from build123d import *

# Parameters (mm, degrees)
F0_W     = 25
F0_H     = 25
F1_DEPTH = 25
F2_W     = 8
F2_H     = 3
F3_DEPTH = 25
F4_W     = 20
F4_H     = 5
F5_DEPTH = 3
F7_DEPTH = 1


with BuildPart() as f1:
    # F0 (on Top) → F1 (new body)
    with BuildSketch(Plane.XY):
        Rectangle(F0_W, F0_H)
    extrude(amount=F1_DEPTH)

    # F2 (on face) → F3 (join)
    with BuildSketch(Plane.XY.offset(25)):
        with Locations((6.7, -1.5)):
            Rectangle(F2_W, F2_H)
        with Locations((-6.7, -1.5)):
            Rectangle(F2_W, F2_H)
    extrude(amount=F3_DEPTH)

    # F4 (on face) → F5 (cut)
    with BuildSketch(Plane.XZ.offset(12.5)):
        with Locations((0, 4.7)):
            Rectangle(F4_W, F4_H)
    extrude(amount=-F5_DEPTH, mode=Mode.SUBTRACT)

    # F6 (on face) → F7 (join)
    with BuildSketch(Plane.XZ.offset(12.5)):
        with BuildLine():
            add(Edge.make_bspline(
                [(-6.6, 15.000625), (-4.434936, 15.000625), (-5.517468, 18.000625), (-6.6, 21.000625), (-7.682532, 18.000625), (-8.765064, 15.000625), (-6.6, 15.000625)],
                knots=[0, 0, 0, 2.094395, 2.094395, 4.18879, 4.18879, 6.283185, 6.283185, 6.283185], degree=2, weights=[1, 0.5, 1, 0.5, 1, 0.5, 1]))
        make_face()
        with BuildLine():
            add(Edge.make_bspline(
                [(6.6, 15.000625), (8.765064, 15.000625), (7.682532, 18.000625), (6.6, 21.000625), (5.517468, 18.000625), (4.434936, 15.000625), (6.6, 15.000625)],
                knots=[0, 0, 0, 2.094395, 2.094395, 4.18879, 4.18879, 6.283185, 6.283185, 6.283185], degree=2, weights=[1, 0.5, 1, 0.5, 1, 0.5, 1]))
        make_face()
    extrude(amount=F7_DEPTH)


solid = f1.part
Source: CAD feature listing. Evaluate the final solid. Frame: model axes, mm. A direction names the side the tool comes from. Round coordinates to 2 decimals unless told otherwise and drop trailing zeros. Loops run counter-clockwise (first coordinate to the right, second up) from the corner with the lowest first, then second, coordinate; pieces in that order, holes last. Notation, with made-up numbers: M 8,69.5 L 52,69.5 A29 cw 52,104.5 Z; hole C -30,41.5 d10. An arc over 180 degrees is marked long. Return JSON: item names as keys, results as strings. Group by question number.
1. Section query B-B on z = 31.5. Output: boundary loops of the cut face in (x, y), and give its area (3 significant figures).
2. Section query A-A on x = -1.5. Output: boundary loops of the cut face in (y, z).
3. Mould query, pull axis Z, two halves, no side actions, for faces 5 (the face through (10, -11, 5)), 6 (the face through (-10.7, -2, 37)), 7 (the face through (0, -11, 7.2)), 8 (the face through (7, -1, 50)). Classes: released by +Z, released by -Z, zero draft, split by the parting line, or undercut.
4. Reachability of faces 1 (the face through (0, -9.5, 5)), 2 (the face through (2.7, -2, 37)), 3 (the face through (7, -3, 37)), 4 (the face through (7, 0, 37)) from +Z, -Z, +X, -X, +Y, -Y: full face, straight path, thin tool, end or side. Return the list, or none.
5. Section query D-D on z = 6. Output: boundary loops of the cut face in (x, y).
6. Pin query (flat end, axial travel): pin 1 (0.9 mm diameter, centred on x = 3.5, y = -11.5, fed in from -Z); pin 2 (3.5 mm diameter, centred on x = 2, y = -11.5, fed in from +Z); pin 3 (4 mm diameter, centred on x = -10, z = 44.5, fed in from -Y); pin 4 (2.5 mm diameter, centred on x = -7, z = 40.5, fed in from +Y). Return the tip coordinate at first contact, or that it passes through.
7. Material intervals for line 1 along X through (y, z) = (-2, 39); line 2 along Z through (x, y) = (3.5, -4.75); line 3 along Y through (x, z) = (-1.75, 13), sorted ascending. Write a range as from..to.
8. Section query C-C on y = -1.25. Output: boundary loops of the cut face in (x, z), and give its area (4 significant figures).
Checks:
{
 "1": {"outline": "M -10.7,-3 L -2.7,-3 L -2.7,0 L -10.7,0 Z; M 2.7,-3 L 10.7,-3 L 10.7,0 L 2.7,0 Z", "area": "48.0 mm²"},
 "2": {"outline": "M -12.5,0 L 12.5,0 L 12.5,25 L -12.5,25 L -12.5,7.2 L -9.5,7.2 L -9.5,2.2 L -12.5,2.2 Z"},
 "3": {"face 5": "undercut", "face 6": "zero draft", "face 7": "undercut", "face 8": "released by +Z"},
 "4": {"face 1": "-Y", "face 2": "+Z, +Y, -Y", "face 3": "+Z, +X, -X, -Y", "face 4": "+Z, +X, -X, +Y"},
 "5": {"outline": "M -12.5,-12.5 L -10,-12.5 L -10,-9.5 L 10,-9.5 L 10,-12.5 L 12.5,-12.5 L 12.5,12.5 L -12.5,12.5 Z"},
 "6": {"pin 1": "stops at z = 0", "pin 2": "stops at z = 25", "pin 3": "stops at y = -3", "pin 4": "stops at y = 0"},
 "7": {"line 1": "x = -10.7..-2.7, 2.7..10.7", "line 2": "z = 0..25", "line 3": "y = -12.5..12.5"},
 "8": {"outline": "M -12.5,0 L 12.5,0 L 12.5,25 L 10.7,25 L 10.7,50 L 2.7,50 L 2.7,25 L -2.7,25 L -2.7,50 L -10.7,50 L -10.7,25 L -12.5,25 Z", "area": "1,025 mm²"}
}
